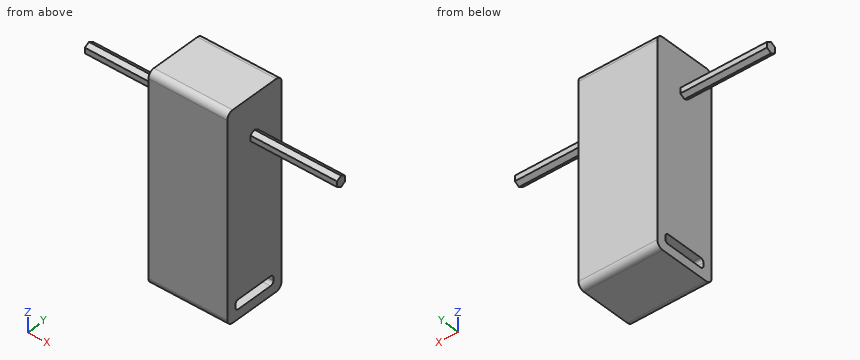
from build123d import *

# Parameters (mm, degrees)
SKETCH_1_W          = 65
SKETCH_1_H          = 20
EXTRUDE_1_DEPTH     = 25
FILLET_1_R          = 2
FILLET_2_R          = 2
FILLET_3_R          = 2
FILLET_4_R          = 2
EXTRUDE_2_DEPTH     = 40
CUT_EXTRUDE_1_DEPTH = 5


with BuildPart() as part:
    # 草图1 → 凸台-拉伸1 (new body)
    with BuildSketch(Plane(origin=(0, 0, 0), x_dir=(0, 0, -1), z_dir=(1, 0, 0))):
        with Locations((0, 10)):
            Rectangle(SKETCH_1_W, SKETCH_1_H)
    extrude(amount=EXTRUDE_1_DEPTH)

    # 圆角1
    fillet_1_edges = [part.edges().sort_by_distance(p)[0] for p in [
        (12.5, 20, 32.5),
    ]]
    fillet(fillet_1_edges, radius=FILLET_1_R)

    # 圆角2
    fillet_2_edges = [part.edges().sort_by_distance(p)[0] for p in [
        (12.5, 0, 32.5),
    ]]
    fillet(fillet_2_edges, radius=FILLET_2_R)

    # 圆角3
    fillet_3_edges = [part.edges().sort_by_distance(p)[0] for p in [
        (12.5, 20, -32.5),
    ]]
    fillet(fillet_3_edges, radius=FILLET_3_R)

    # 圆角4
    fillet_4_edges = [part.edges().sort_by_distance(p)[0] for p in [
        (12.5, 0, -32.5),
    ]]
    fillet(fillet_4_edges, radius=FILLET_4_R)

    # 草图3 → 凸台-拉伸2 (add, symmetric)
    with BuildSketch(Plane.ZY.offset(-12.5)):
        Polygon((18.267949192, 10), (19.133974596, 8.5), (20.866025404, 8.5), (21.732050808, 10), (20.866025404, 11.5), (19.133974596, 11.5), align=None)
    extrude(amount=EXTRUDE_2_DEPTH, both=True)

    # 草图4 → 切除-拉伸1 (cut)
    with BuildSketch(Plane.ZY.offset(-25)):
        with BuildLine():
            Line((-29.5, 4), (-29.5, 16))
            ThreePointArc((-29.5, 16), (-29.207106781, 16.707106781), (-28.5, 17))
            Line((-28.5, 17), (-27.5, 17))
            ThreePointArc((-27.5, 17), (-26.792893219, 16.707106781), (-26.5, 16))
            Line((-26.5, 16), (-26.5, 4))
            ThreePointArc((-26.5, 4), (-26.792893219, 3.292893219), (-27.5, 3))
            Line((-27.5, 3), (-28.5, 3))
            ThreePointArc((-28.5, 3), (-29.207106781, 3.292893219), (-29.5, 4))
        make_face()
    cut_extrude_1 = extrude(amount=CUT_EXTRUDE_1_DEPTH, mode=Mode.SUBTRACT)

    # 镜向1: 切除-拉伸1 across plane
    add(cut_extrude_1.mirror(Plane.ZY.offset(-12.5)), mode=Mode.SUBTRACT)


solid = part.part
Geometry: final body of the model. Coordinates: model frame, mm. Coordinates: 2 decimals unless noted, no trailing zeros. Loops run counter-clockwise (first coordinate to the right, second up) from the corner with the lowest first, then second, coordinate; pieces in that order, holes last. Notation, with made-up numbers: M 30,-40 L 44,-40 A30 cw 44,-9 Z; hole C 78,15 d9. An arc over 180 degrees is marked long. One line per item, written item: value. Start each with the question number.
1) Cut plane A-A (y = 13.75). Return loops of the section in (x, z), then the cut area to 4 significant figures.
2) Material intervals for L1, parallel to X at y = 10.25, z = -4.5; L2, parallel to Z at x = 4.5, y = 4.5; L3, parallel to X at y = 10.5, z = -28, sorted ascending. Write a range as from..to.
3) Cut plane C-C (z = -25). Return loops of the section in (x, y), then the cut area to 3 significant figures.
4) Pin query (flat end, axial travel): P1, Ø10, axis at y = 7.5, z = -1.5, coming from the -X side; P2, Ø6, axis at y = 10.5, z = 5, coming from the +X side; P3, Ø0.5, axis at x = 36, z = 19.5, coming from the -Y side. Return the tip coordinate at first contact, or that it passes through.
5) Cut plane B-B (x = 35). Return loops of the section in (y, z), then the cut area to 3 significant figures.
Evaluation:
1. outline: M 0,-32.5 L 25,-32.5 L 25,-29.5 L 20,-29.5 L 20,-26.5 L 25,-26.5 L 25,32.5 L 0,32.5 L 0,-26.5 L 5,-26.5 L 5,-29.5 L 0,-29.5 Z
1. area: 1,595 mm^2
2. L1: 0..25
2. L2: -32.5..-29.5, -26.5..32.5
2. L3: 5..20
3. outline: M 0,0 L 25,0 L 25,20 L 0,20 Z
3. area: 500 mm^2
4. P1: x = 0
4. P2: x = 25
4. P3: y = 8.5
5. outline: M 8.5,19.13 L 10,18.27 L 11.5,19.13 L 11.5,20.87 L 10,21.73 L 8.5,20.87 Z
5. area: 7.79 mm^2
